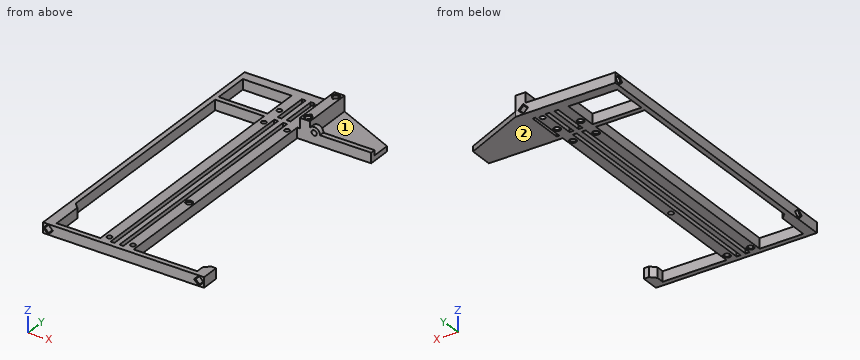
from build123d import *

# Parameters (mm, degrees)
BOSS_EXTRUDE1_START                    = -9.525
SKETCH1_W                              = 2.158991534
SKETCH1_H                              = 29.633333333
SKETCH1_W_2                            = 40.548965045
SKETCH1_W_3                            = 3.220517478
SKETCH1_W_4                            = 3.220517477
SKETCH1_H_2                            = 201.083333334
BOSS_EXTRUDE1_DEPTH                    = 8.466666667
BOSS_EXTRUDE2_DEPTH                    = 4.318
SKETCH16_W                             = 8.466666666
SKETCH16_H                             = 42.333333333
BOSS_EXTRUDE3_DEPTH                    = 8.466666667
SKETCH18_R                             = 4.7625
BOSS_EXTRUDE4_DEPTH                    = 4.233333333
F_18_0_1695_DIAMETER_HOLE3_D           = 4.3053
F_18_0_1695_DIAMETER_HOLE3_DEPTH       = 4.233333333
F_18_0_1695_DIAMETER_HOLE1_D           = 4.3053
F_18_0_1695_DIAMETER_HOLE1_CSINK_D     = 5.5753
F_18_0_1695_DIAMETER_HOLE1_CSINK_ANGLE = 90
BOTTOM_PINS_DEPTH                      = 6.35
REAR_PINS_DEPTH                        = 6.35
LEFT_PINS_DEPTH                        = 6.35
CUT_EXTRUDE3_DEPTH                     = 6.35
CHAMFER2_SIZE                          = 0.635
F_18_0_1695_DIAMETER_HOLE2_D           = 4.3053
F_18_0_1695_DIAMETER_HOLE2_DEPTH       = 8.382
F_18_0_1695_DIAMETER_HOLE2_CSINK_D     = 5.5753
F_18_0_1695_DIAMETER_HOLE2_CSINK_ANGLE = 90
F_18_0_1695_DIAMETER_HOLE2_TIP         = 1.293442612


with BuildPart() as part:
    # Sketch1 → Boss-Extrude1 (new body)
    with BuildSketch(Plane.XY.offset(BOSS_EXTRUDE1_START)):
        Polygon((47.413333333, 127), (130.428991533, 127), (130.428991533, 88.9), (181.228991533, 88.9), (181.228991533, 84.666666667), (119.803333333, 84.666666667), (119.803333333, -116.416666667), (172.762324867, -116.416666667), (172.762324867, -110.066666667), (176.9956582, -105.833333333), (181.228991533, -105.833333333), (181.228991533, -120.65), (47.413333333, -120.65), align=None)
        with Locations((120.8828291, 103.716666667)):
            Rectangle(SKETCH1_W, SKETCH1_H, mode=Mode.SUBTRACT)
        Polygon((55.88, -116.416666667), (55.88, -91.016666667), (51.646666667, -86.783333333), (51.646666667, 84.666666667), (92.195631712, 84.666666667), (92.195631712, -116.416666667), align=None, mode=Mode.SUBTRACT)
        with Locations((71.921149189, 103.716666667)):
            Rectangle(SKETCH1_W_2, SKETCH1_H, mode=Mode.SUBTRACT)
        with Locations((109.726407928, 103.716666667)):
            Rectangle(SKETCH1_W_3, SKETCH1_H, mode=Mode.SUBTRACT)
        with Locations((102.272557118, -15.875)):
            Rectangle(SKETCH1_W_4, SKETCH1_H_2, mode=Mode.SUBTRACT)
        with Locations((102.272557118, 103.716666667)):
            Rectangle(SKETCH1_W_4, SKETCH1_H, mode=Mode.SUBTRACT)
        with Locations((109.726407928, -15.875)):
            Rectangle(SKETCH1_W_3, SKETCH1_H_2, mode=Mode.SUBTRACT)
    extrude(amount=-BOSS_EXTRUDE1_DEPTH)

    # Sketch9 → Boss-Extrude2 (add)
    with BuildSketch(Plane.XY.offset(-17.991666667)):
        Polygon((181.228991533, 88.9), (130.428991533, 88.9), (130.428991533, 127), (181.228991533, 104.14), align=None)
    extrude(amount=BOSS_EXTRUDE2_DEPTH)

    # Sketch16 → Boss-Extrude3 (add)
    with BuildSketch(Plane.XY.offset(-9.525)):
        with Locations((126.1956582, 105.833333334)):
            Rectangle(SKETCH16_W, SKETCH16_H)
    extrude(amount=BOSS_EXTRUDE3_DEPTH)

    # Sketch18 → Boss-Extrude4 (add)
    with BuildSketch(Plane(origin=(0, 84.666666667, 0), x_dir=(-1, 0, 0), z_dir=(0, -1, 0))):
        with Locations((-133.889, 9.251666559)):
            Circle(SKETCH18_R)
    extrude(amount=-BOSS_EXTRUDE4_DEPTH)

    # #18 (0.1695) Diameter Hole3
    with Locations(Plane(origin=(0, 88.9, 0), x_dir=(1, 0, 0), z_dir=(0, 1, 0))):
        with Locations((133.889, 9.251666559)):
            Hole(F_18_0_1695_DIAMETER_HOLE3_D / 2, depth=F_18_0_1695_DIAMETER_HOLE3_DEPTH)

    # #18 (0.1695) Diameter Hole1 (through all)
    with Locations(Plane.XY.offset(-9.525)):
        with Locations((115.57, 115.57), (115.57, -41.91)):
            CounterSinkHole(F_18_0_1695_DIAMETER_HOLE1_D / 2, F_18_0_1695_DIAMETER_HOLE1_CSINK_D / 2, counter_sink_angle=F_18_0_1695_DIAMETER_HOLE1_CSINK_ANGLE)

    # Sketch2 → bottom pins (cut)
    with BuildSketch(Plane.XZ.offset(120.65)):
        Polygon((173.8206582, -13.758333333), (176.9956582, -10.583333333), (180.1706582, -13.758333333), (176.9956582, -16.933333333), align=None)
        Polygon((48.471666667, -13.758333333), (51.646666667, -10.583333333), (54.821666667, -13.758333333), (51.646666667, -16.933333333), align=None)
    extrude(amount=-BOTTOM_PINS_DEPTH, mode=Mode.SUBTRACT)

    # Sketch3 → rear pins (cut)
    with BuildSketch(Plane.ZY.offset(-47.413333333)):
        Polygon((-16.933333333, 122.766666667), (-13.758333333, 125.941666667), (-10.583333333, 122.766666667), (-13.758333333, 119.591666667), align=None)
        Polygon((-16.933333333, -97.79), (-13.758333333, -94.615), (-10.583333333, -97.79), (-13.758333333, -100.965), align=None)
    extrude(amount=-REAR_PINS_DEPTH, mode=Mode.SUBTRACT)

    # Sketch8 → left pins (cut)
    with BuildSketch(Plane.XY.offset(-1.058333333)):
        Polygon((123.0206582, 88.9), (126.1956582, 92.075), (129.3706582, 88.9), (126.1956582, 85.725), align=None)
        Polygon((123.0206582, 122.766666667), (126.1956582, 125.941666667), (129.3706582, 122.766666667), (126.1956582, 119.591666667), align=None)
    extrude(amount=-LEFT_PINS_DEPTH, mode=Mode.SUBTRACT)

    # Sketch24 → Cut-Extrude3 (cut)
    with BuildSketch(Plane(origin=(0, 127, 0), x_dir=(1, 0, 0), z_dir=(0, 1, 0))):
        Polygon((120.903991533, 13.758333333), (124.078991533, 16.933333333), (127.253991533, 13.758333333), (124.078991533, 10.583333333), align=None)
    extrude(amount=-CUT_EXTRUDE3_DEPTH, mode=Mode.SUBTRACT)

    # Chamfer2
    chamfer2_edges = [part.edges().sort_by_distance(p)[0] for p in [
        (175.4081582, -114.3, -15.345833333),
        (175.4081582, -114.3, -12.170833333),
        (178.5831582, -114.3, -12.170833333),
        (178.5831582, -114.3, -15.345833333),
        (175.4081582, -120.65, -15.345833333),
        (178.5831582, -120.65, -15.345833333),
        (178.5831582, -120.65, -12.170833333),
        (175.4081582, -120.65, -12.170833333),
        (50.059166667, -114.3, -15.345833333),
        (50.059166667, -114.3, -12.170833333),
        (53.234166667, -114.3, -12.170833333),
        (53.234166667, -114.3, -15.345833333),
        (50.059166667, -120.65, -15.345833333),
        (53.234166667, -120.65, -15.345833333),
        (53.234166667, -120.65, -12.170833333),
        (50.059166667, -120.65, -12.170833333),
        (53.763333333, 121.179166667, -15.345833333),
        (53.763333333, 124.354166667, -15.345833333),
        (53.763333333, 124.354166667, -12.170833333),
        (53.763333333, 121.179166667, -12.170833333),
        (47.413333333, 121.179166667, -15.345833333),
        (47.413333333, 121.179166667, -12.170833333),
        (47.413333333, 124.354166667, -12.170833333),
        (47.413333333, 124.354166667, -15.345833333),
        (53.763333333, -99.3775, -15.345833333),
        (53.763333333, -96.2025, -15.345833333),
        (53.763333333, -96.2025, -12.170833333),
        (53.763333333, -99.3775, -12.170833333),
        (47.413333333, -99.3775, -15.345833333),
        (47.413333333, -99.3775, -12.170833333),
        (47.413333333, -96.2025, -12.170833333),
        (47.413333333, -96.2025, -15.345833333),
        (124.6081582, 87.3125, -7.408333333),
        (124.6081582, 90.4875, -7.408333333),
        (127.7831582, 90.4875, -7.408333333),
        (127.7831582, 87.3125, -7.408333333),
        (124.6081582, 87.3125, -1.058333333),
        (127.7831582, 87.3125, -1.058333333),
        (127.7831582, 90.4875, -1.058333333),
        (124.6081582, 90.4875, -1.058333333),
        (124.6081582, 121.179166667, -7.408333333),
        (124.6081582, 124.354166667, -7.408333333),
        (127.7831582, 124.354166667, -7.408333333),
        (127.7831582, 121.179166667, -7.408333333),
        (124.6081582, 121.179166667, -1.058333333),
        (127.7831582, 121.179166667, -1.058333333),
        (127.7831582, 124.354166667, -1.058333333),
        (124.6081582, 124.354166667, -1.058333333),
        (122.491491533, 120.65, -12.170833333),
        (122.491491533, 120.65, -15.345833333),
        (125.666491533, 120.65, -15.345833333),
        (125.666491533, 120.65, -12.170833333),
        (122.491491533, 127, -12.170833333),
        (125.666491533, 127, -12.170833333),
        (125.666491533, 127, -15.345833333),
        (122.491491533, 127, -15.345833333),
    ]]
    chamfer(chamfer2_edges, length=CHAMFER2_SIZE)

    # #18 (0.1695) Diameter Hole2
    with Locations(Plane(origin=(0, 0, -17.991666667), x_dir=(-1, 0, 0), z_dir=(0, 0, -1))):
        with Locations((-116.077975238, 97.155), (-96.527983128, 97.155), (-96.727984128, 77.805001), (-116.077983128, 77.605), (-116.077983128, -111.625), (-96.527983128, -111.625)):
            CounterSinkHole(F_18_0_1695_DIAMETER_HOLE2_D / 2, F_18_0_1695_DIAMETER_HOLE2_CSINK_D / 2, depth=F_18_0_1695_DIAMETER_HOLE2_DEPTH, counter_sink_angle=F_18_0_1695_DIAMETER_HOLE2_CSINK_ANGLE)
            with Locations((0, 0, -(F_18_0_1695_DIAMETER_HOLE2_DEPTH + F_18_0_1695_DIAMETER_HOLE2_TIP / 2))):  # 118° drill point
                Cone(0, F_18_0_1695_DIAMETER_HOLE2_D / 2, F_18_0_1695_DIAMETER_HOLE2_TIP, mode=Mode.SUBTRACT)


solid = part.part
Geometry: final body of the model. Coordinates: model frame, mm. Face numbers are marked on the shaded views. A direction names the side the tool comes from. Give positions to 0.01 mm unless a question says otherwise; leave off trailing zeros. Write each loop counter-clockwise with the first axis right and the second up, starting at its lowest first coordinate (ties: lowest second). Pieces come first, ordered by that corner, then holes.
(1) First-contact query: P1, Ø2, axis at x = 154, z = -8, coming from the +Y side; P2, Ø3, axis at y = 96.5, z = -11, coming from the +X side; P3, Ø3.5, axis at x = 126, y = 124, coming from the +Z side; P4, Ø7, axis at y = -10.5, z = -15.5, coming from the +X side. Flat tips, straight axial feed; report the tip coordinate or a pass-through.
(2) Cut plane B-B, the plane x = 69. Return loops of the section in (y, z) (3 decimals), then the cut area to 3 significant figures.
(3) Cut plane C-C, the plane x = 167. Return loops of the section in (y, z) (3 decimals), then the cut area to 3 significant figures.
(4) Access query for the marked faces 1 and 2. Directions: +Z, -Z, +X, -X, +Y, -Y. A direction counts if a zero-diameter tool reaches every point of the face in a straight line with its end or side. Return the directions, or none.
(5) Cut plane A-A, the plane y = 39.5. Return loops of the section in (x, z) (3 decimals), then the cut area to 3 significant figures.
(6) Ray query, line 1 (X direction, y = -41.91, z = -14); line 2 (Y direction, x = 61.5, z = -16); line 3 (X direction, y = 25.5, z = -15). Return the intervals inside material, ascending.
Values follow:
1. P1: passes through
1. P2: stops at x = 130.43
1. P3: stops at z = -1.18
1. P4: stops at x = 119.8
2. outline: (-120.65, -17.992) - (-116.417, -17.992) - (-116.417, -9.525) - (-120.65, -9.525) - close; (84.667, -17.992) - (88.9, -17.992) - (88.9, -9.525) - (84.667, -9.525) - close; (118.533, -17.992) - (127, -17.992) - (127, -9.525) - (118.533, -9.525) - close
2. area: 143 mm2
3. outline: (-120.65, -17.992) - (-116.417, -17.992) - (-116.417, -9.525) - (-120.65, -9.525) - close; (84.667, -17.992) - (110.543, -17.992) - (110.543, -13.674) - (88.9, -13.674) - (88.9, -9.525) - (84.667, -9.525) - close
3. area: 165 mm2
4. face 1: +Z, +X, +Y
4. face 2: -Z, +X, -X, +Y, -Y
5. outline: (47.413, -17.992) - (51.647, -17.992) - (51.647, -9.525) - (47.413, -9.525) - close; (92.196, -17.992) - (100.662, -17.992) - (100.662, -9.525) - (92.196, -9.525) - close; (103.883, -17.992) - (108.116, -17.992) - (108.116, -9.525) - (103.883, -9.525) - close; (111.337, -17.992) - (119.803, -17.992) - (119.803, -9.525) - (111.337, -9.525) - close
5. area: 215 mm2
6. line 1: x = 47.41 to 51.65, 92.2 to 100.66, 103.88 to 108.12, 111.34 to 113.42, 117.72 to 119.8
6. line 2: y = -120.65 to -116.42, 84.67 to 88.9, 118.53 to 127
6. line 3: x = 47.41 to 51.65, 92.2 to 100.66, 103.88 to 108.12, 111.34 to 119.8
